Read the model definition and answer for the solid it produces. Units are mm, in the model's axes. A direction names the side the tool comes from. Coordinates: 2 decimals unless noted, no trailing zeros. Write each loop counter-clockwise with the first axis right and the second up, starting at its lowest first coordinate (ties: lowest second). Pieces come first, ordered by that corner, then holes. Notation, with made-up numbers: (63.25, 66) -> (121.25, 66) arc R25 ccw to (121.25, 94) -> close; hole circle Ø7 at (21, 74.25). An arc over 180 degrees is marked (long way). Return JSON: item names as keys, results as strings.
from build123d import *

# Parameters (mm, degrees)
F1_DEPTH     = 7.1
F2_W         = 1.45
F2_H         = 0.1
F3_DEPTH     = 0.6
F5_DEPTH     = 1.45
F6_R         = 0.1
F8_DEPTH     = 40
F10_DEPTH    = 3
F11_T1_DEPTH = 3
F11_T3_DEPTH = 4


# Not quite as in the source:
# - a fillet or chamfer that OpenCascade refuses, or shapes differently, is made with other operations: its cross-section is extruded or revolved along the edge and cut away or added


with BuildPart() as f1:
    # F0 (on Front) → F1 (new body)
    with BuildSketch(Plane.XZ):
        with BuildLine():
            Line((-1, 1.8466185313), (-1, 1.9595917942))
            ThreePointArc((-1, 1.9595917942), (0, -2.2), (1, 1.9595917942))
            Line((1, 1.9595917942), (1, 1.8466185313))
            ThreePointArc((1, 1.8466185313), (0, -2.1), (-1, 1.8466185313))
        make_face()
    extrude(amount=F1_DEPTH)

    # F2 (on face) → F3 (join)
    with BuildSketch(Plane(origin=(0, 0, 0), x_dir=(-1, 0, 0), z_dir=(0, 1, 0))):
        with Locations((0, -2.15)):
            Rectangle(F2_W, F2_H)
    extrude(amount=F3_DEPTH)

    # F4 (on face) → F5 (join, through all)
    with BuildSketch(Plane(origin=(-0.725, 0, 0), x_dir=(0, -1, 0), z_dir=(-1, 0, 0))):
        Polygon((-0.6, -3.4), (-0.6, -2.1), (-0.7, -2.1), (-0.7, -3.3), (-7.5, -3.3), (-7.5, -2.9), (-7.5, -2.1), (-12.5, -2.1), (-12.5, -2.9), (-7.6, -2.9), (-7.6, -3.4), align=None)
    extrude(amount=-F5_DEPTH)

    # F6
    f6_edges = [f1.edges().sort_by_distance(p)[0] for p in [
        (0, 0.7, -2.1),
        (0, 0.6, -2.2),
        (0, 0.6, -3.4),
        (0, 0.7, -3.3),
        (0, 7.5, -3.3),
        (0, 7.5, -2.1),
        (0, 7.6, -3.4),
    ]]
    fillet(f6_edges, radius=F6_R)

    # F7 (on Right) → F8 (cut, symmetric)
    with BuildSketch(Plane.YZ):
        Polygon((-4.7, -1.49), (-4.1, 1.9595917942), (-7.1, 1.9595917942), (-7.1, -1.49), align=None)
    extrude(amount=F8_DEPTH, both=True, mode=Mode.SUBTRACT)

    # F9 (on face) → F10 (join)
    with BuildSketch(Plane.XZ.offset(7.1)):
        Polygon((-0.95, 0.6), (-0.95, -2.2), (0.95, -2.2), (0.95, 0.6), (0.85, 0.6), (0.85, -2.1), (-0.85, -2.1), (-0.85, 0.6), align=None)
    extrude(amount=F10_DEPTH)

    # F11: fillet of radius 0.2 on 4 edges, made by hand

    # F11_s2 → F11_t1 (join)
    with BuildSketch(Plane.XZ.offset(7.1)):
        with BuildLine():
            ThreePointArc((-0.85, -1.9), (-0.7914213562, -2.0414213562), (-0.65, -2.1))
            Line((-0.65, -2.1), (-0.85, -2.1))
            Line((-0.85, -2.1), (-0.85, -1.9))
        make_face()
        with BuildLine():
            ThreePointArc((0.65, -2.1), (0.7914213562, -2.0414213562), (0.85, -1.9))
            Line((0.85, -1.9), (0.85, -2.1))
            Line((0.85, -2.1), (0.65, -2.1))
        make_face()
    extrude(amount=F11_T1_DEPTH)

    # F11_s4 → F11_t3 (cut)
    with BuildSketch(Plane.XZ.offset(6.6)):
        with BuildLine():
            ThreePointArc((-0.95, -2), (-0.8914213562, -2.1414213562), (-0.75, -2.2))
            Line((-0.75, -2.2), (-0.95, -2.2))
            Line((-0.95, -2.2), (-0.95, -2))
        make_face()
        with BuildLine():
            ThreePointArc((0.95, -2), (0.8914213562, -2.1414213562), (0.75, -2.2))
            Line((0.75, -2.2), (0.95, -2.2))
            Line((0.95, -2.2), (0.95, -2))
        make_face()
    extrude(amount=F11_T3_DEPTH, mode=Mode.SUBTRACT)


solid = f1.part
1. The part is cut by section A-A (z = 0). Determine the outline of the cut face in (x, y), then the cut area to 3 significant figures.
Taken from the geometry:
{"outline": "(-2.2, -4.44) -> (-2.1, -4.44) -> (-2.1, 0) -> (-2.2, 0) -> close; (-0.95, -10.1) -> (-0.85, -10.1) -> (-0.85, -7.1) -> (-0.95, -7.1) -> close; (0.85, -10.1) -> (0.95, -10.1) -> (0.95, -7.1) -> (0.85, -7.1) -> close; (2.1, -4.44) -> (2.2, -4.44) -> (2.2, 0) -> (2.1, 0) -> close", "area": "1.49 mm2"}
2. The part is cut by section B-B (y = -3.25). Determine the outline of the cut face in (x, z).
Taken from the geometry:
{"outline": "(-1, 1.85) -> (-1, 1.96) arc R2.2 ccw (long way) to (1, 1.96) -> (1, 1.85) arc R2.1 cw (long way) to start"}
3. Flat-ended cylindrical pins translate along their axes: pin 1 Ø1.2 at (y, z) = (-9.5, -0.5) entering from +X; pin 2 Ø2.5 at (x, z) = (-1, 0.5) entering from +Y; pin 3 Ø1.6 at (x, y) = (0, 10) entering from -Z. Find the tip coordinate at first contact, or state that the pin passes through.
Taken from the geometry:
{"pin 1": "stops at x = 0.95", "pin 2": "stops at y = 0", "pin 3": "stops at z = -2.9"}
4. A tool of negligible diameter and unlimited length cuts with its end or side. For faces 1 (the face through (0, 10, -2.1)), 2 (the face through (0, 10, -2.9)), 3 (the face through (0, 7.5, -2.7)), from which of +Z, -Z, +X, -X, +Y, -Y can it reach the whole face along a straight path? Write none if from no direction.
Taken from the geometry:
{"face 1": "+Z, +X, -X, +Y", "face 2": "-Z, +X, -X, +Y", "face 3": "+Z, +X, -X"}
5. The part is cut by section D-D (y = 1). Determine the outline of the cut face in (x, z) (3 decimals).
Taken from the geometry:
{"outline": "(-0.725, -3.4) -> (0.725, -3.4) -> (0.725, -3.3) -> (-0.725, -3.3) -> close"}
